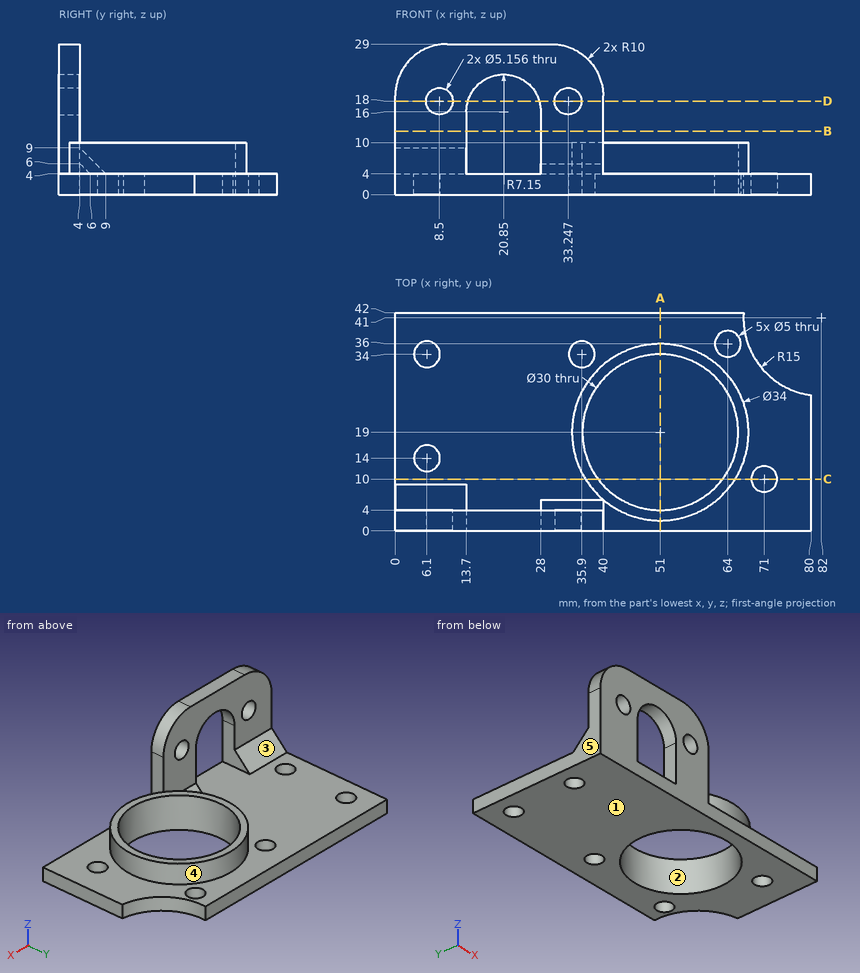
Job drawing, mm, ordinate dimensions from the low corner. One solid piece. A direction names the side the tool comes from. Coordinates: 2 decimals unless noted, no trailing zeros. Write each loop counter-clockwise with the first axis right and the second up, starting at its lowest first coordinate (ties: lowest second). Pieces come first, ordered by that corner, then holes. Notation, with made-up numbers: M 34.25,-31 L 48.25,-31 A23 ccw 48.25,1 Z; hole C 55,20 d3. An arc over 180 degrees is marked long. Answer as a JSON object with one key per item and string values. Group by question number.
1) Saw through at A-A (x = 51). Write the cut outline in (y, z).
2) Mould opens along Y. For the marked faces 1, 2 and 3 say: +Y half, -Y half, draft (parallel to the pull), parting line (faces both ways), or undercut.
3) Saw through at D-D (z = 18). Write the cut outline in (x, y) (1 decimal).
4) Pin check, flat tips, straight feed: pin 1 Ø2.5 at (y, z) = (2.5, 13) entering from +X; pin 2 Ø10 at (x, z) = (36, 18.5) entering from +Y. Stop position of each tip, or through.
5) Wall check: line 1 (Y direction, x = 6.1, z = 1.6); line 2 (X direction, y = 2.55, z = 18) (1 decimal); line 3 (X direction, y = 3, z = 10.75). Give the ranges that are in metal, low to high. Write a range as from..to.
6) Tool access for the marked faces 4 and 5: list every direction of +Z, -Z, +X, -X, +Y, -Y with a clear straight run to the whole face (end or side of a thin tool).
7) Saw through at C-C (y = 10). Write the cut outline in (x, z), plus the area to 3 significant figures.
8) Saw through at B-B (z = 12.25). Write the cut outline in (x, y), plus the area to 3 significant figures.
Values follow:
{
 "1": {"outline": "M 0,0 L 4,0 L 4,10 L 2,10 L 2,4 L 0,4 Z; M 34,0 L 42,0 L 42,4 L 36,4 L 36,10 L 34,10 Z"},
 "2": {"face 1": "draft", "face 2": "undercut", "face 3": "+Y half"},
 "3": {"outline": "M 0,0 L 5.9,0 L 5.9,4 L 0,4 Z; M 11.1,0 L 14,0 L 14,4 L 11.1,4 Z; M 27.7,0 L 30.7,0 L 30.7,4 L 27.7,4 Z; M 35.8,0 L 40,0 L 40,4 L 35.8,4 Z"},
 "4": {"pin 1": "stops at x = 40", "pin 2": "stops at y = 4"},
 "5": {"line 1": "y = 0..11.5, 16.5..31.5, 36.5..42", "line 2": "x = 0..5.9, 11.1..14, 27.7..30.7, 35.8..40", "line 3": "x = 0..13.7, 28..40"},
 "6": {"face 4": "+Z", "face 5": "+Z, -Z, -X, +Y, -Y"},
 "7": {"outline": "M 0,0 L 39,0 L 39,10 L 36.58,10 L 36.58,4 L 0,4 Z; M 63,0 L 68.5,0 L 68.5,4 L 65.42,4 L 65.42,10 L 63,10 Z; M 73.5,0 L 80,0 L 80,4 L 73.5,4 Z", "area": "233 mm2"},
 "8": {"outline": "M 0,0 L 13.7,0 L 13.7,4 L 0,4 Z; M 28,0 L 40,0 L 40,4 L 28,4 Z", "area": "103 mm2"}
}
